Work out the finished part from the listing and answer in its coordinate system (mm). A direction names the side the tool comes from. Give positions to 0.01 mm unless a question says otherwise; leave off trailing zeros. Write each loop counter-clockwise with the first axis right and the second up, starting at its lowest first coordinate (ties: lowest second). Pieces come first, ordered by that corner, then holes.
1) Determine the mould class of faces 5 (the face through (20.35, 0, -14)), 6 (the face through (16, 5, 0.5)), 7 (the face through (0.1, -7, 0.5)) for opening direction Y: pulls with the +Y half, pulls with the -Y half, needs draft (parallel to the pull), parting line crosses it, or undercut.
2) A tool of negligible diameter and unlimited length cuts with its end or side. For faces 1 (the face through (19.065, 0.07, -0.301)), 2 (the face through (-16, -5, 0.5)), 3 (the face through (15.8, -5, 0.5)), 4 (the face through (-10.5, -1.5, 0.5)), from which of +Z, -Z, +X, -X, +Y, -Y can it reach the whole face along a straight path? Write none if from no direction.
3) Find section A-A (z = -5.5). Determine the outline of the cut face in (x, y), plus the area to 3 significant figures.
4) Find section B-B (y = 0). Count the separate pieces of the cut face and the enclosed holes in it, plus the area to 3 significant figures.
5) Find section D-D (x = -5). Determine the outline of the cut face in (y, z).
6) Straight lines are drawn through the part: probe 1 along Y at (x, z) = (20, -25); probe 2 along X at (y, z) = (1.75, -18.75); probe 3 along Z at (x, y) = (4.5, 9). For each, find the intervals that lie inside material, in ascending order.
7) Given pin 1 Ø3.5 at (x, y) = (0, 0) entering from +Z; pin 2 Ø0.8 at (x, z) = (-15.5, 0.5) entering from +Y; pin 3 Ø4 at (y, z) = (0, -25) entering from -X; pin 4 Ø3 at (x, y) = (-1, -7.5) entering from -Z, each flat-ended and moving along its own axis, determine where each tip first touches the part or whether it passes through.
8) Find section C-C (x = 0). Determine the outline of the cut face in (y, z).
```python
from build123d import *

# Parameters (mm, degrees)
SKETCH1_R           = 3
BOSS_EXTRUDE1_DEPTH = 1
SKETCH2_R           = 1.3
BOSS_EXTRUDE2_DEPTH = 1
FILLET1_R           = 1
CUT_EXTRUDE1_DEPTH  = 1


with BuildPart() as part:
    # Sketch1 → Boss-Extrude1 (new body)
    with BuildSketch(Plane.XY):
        with BuildLine():
            ThreePointArc((11.456439237, 5), (0, 12.5), (-11.456439237, 5))
            Line((-11.456439237, 5), (11.456439237, 5))
        make_face()
        with BuildLine():
            Line((11.456439237, 5), (-11.456439237, 5))
            ThreePointArc((-11.456439237, 5), (-12.5, 0), (-11.456439237, -5))
            Line((-11.456439237, -5), (11.456439237, -5))
            ThreePointArc((11.456439237, -5), (12.236328912, -2.553870546), (12.5, 0))
            ThreePointArc((12.5, 0), (12.236328912, 2.553870546), (11.456439237, 5))
        make_face()
        Circle(SKETCH1_R, mode=Mode.SUBTRACT)
        with BuildLine():
            Line((20.35, 5), (11.456439237, 5))
            ThreePointArc((11.456439237, 5), (12.236328912, 2.553870546), (12.5, 0))
            ThreePointArc((12.5, 0), (12.236328912, -2.553870546), (11.456439237, -5))
            Line((11.456439237, -5), (20.35, -5))
            Line((20.35, -5), (20.35, 5))
        make_face()
        with BuildLine():
            Line((-11.456439237, 5), (-20.35, 5))
            Line((-20.35, 5), (-20.35, -5))
            Line((-20.35, -5), (-11.456439237, -5))
            ThreePointArc((-11.456439237, -5), (-12.5, 0), (-11.456439237, 5))
        make_face()
        with BuildLine():
            Line((11.456439237, -5), (-11.456439237, -5))
            ThreePointArc((-11.456439237, -5), (0, -12.5), (11.456439237, -5))
        make_face()
    extrude(amount=BOSS_EXTRUDE1_DEPTH)

    # Sketch2 → Boss-Extrude2 (add)
    with BuildSketch(Plane.ZY.offset(20.35)):
        with BuildLine():
            Line((-25, -3), (0, -5))
            Line((0, -5), (0, 5))
            Line((0, 5), (-25, 3))
            ThreePointArc((-25, 3), (-28, 0), (-25, -3))
        make_face()
        with Locations((-25, 0)):
            Circle(SKETCH2_R, mode=Mode.SUBTRACT)
    boss_extrude2 = extrude(amount=-BOSS_EXTRUDE2_DEPTH)

    # Mirror1: Boss-Extrude2 across plane
    add(boss_extrude2.mirror(Plane.ZY))

    # Fillet1
    fillet1_edges = [part.edges().sort_by_distance(p)[0] for p in [
        (20.35, 0, 1),
        (-20.35, 0, 1),
        (19.35, 0, 0),
        (-19.35, 0, 0),
    ]]
    fillet(fillet1_edges, radius=FILLET1_R)

    # Sketch3 → Cut-Extrude1 (cut)
    with BuildSketch(Plane.XY.offset(1)):
        with BuildLine():
            ThreePointArc((8, 1.5), (6.5, 0), (8, -1.5))
            Line((8, -1.5), (13, -1.5))
            ThreePointArc((13, -1.5), (14.5, 0), (13, 1.5))
            Line((13, 1.5), (8, 1.5))
        make_face()
        with BuildLine():
            ThreePointArc((-4.117647107, 5.660828765), (-1.9e-08, 7), (4.117647076, 5.660828787))
            ThreePointArc((4.117647076, 5.660828787), (6.213034752, 5.991510614), (5.882352933, 8.086898291))
            ThreePointArc((5.882352933, 8.086898291), (6e-09, 10), (-5.882352923, 8.086898298))
            ThreePointArc((-5.882352923, 8.086898298), (-6.213034767, 5.991510634), (-4.117647107, 5.660828765))
        make_face()
        with BuildLine():
            ThreePointArc((4.117647035, -5.660828817), (-2.5e-08, -7), (-4.117647076, -5.660828787))
            ThreePointArc((-4.117647076, -5.660828787), (-6.213034774, -5.991510645), (-5.882352871, -8.086898336))
            ThreePointArc((-5.882352871, -8.086898336), (7.8e-08, -10), (5.882352997, -8.086898245))
            ThreePointArc((5.882352997, -8.086898245), (6.213034714, -5.991510562), (4.117647035, -5.660828817))
        make_face()
        with BuildLine():
            ThreePointArc((-8, -1.5), (-6.5, 0), (-8, 1.5))
            Line((-8, 1.5), (-13, 1.5))
            ThreePointArc((-13, 1.5), (-14.5, 0), (-13, -1.5))
            Line((-13, -1.5), (-8, -1.5))
        make_face()
    extrude(amount=-CUT_EXTRUDE1_DEPTH, mode=Mode.SUBTRACT)


solid = part.part
```
Results:
1. face 5: needs draft
1. face 6: pulls with the +Y half
1. face 7: undercut
2. face 1: -Z, +Y, -Y
2. face 2: +Z, -Z, -X, -Y
2. face 3: +Z, -Z, +X, -Y
2. face 4: +Z, -Z
3. outline: (-20.35, -4.56) - (-19.35, -4.56) - (-19.35, 4.56) - (-20.35, 4.56) - close; (19.35, -4.56) - (20.35, -4.56) - (20.35, 4.56) - (19.35, 4.56) - close
3. area: 18.2 mm2
4. separate pieces: 6
4. enclosed holes: 0
4. area: 69.5 mm2
5. outline: (-11.46, 0) - (-8.66, 0) - (-8.66, 1) - (-11.46, 1) - close; (-5.37, 0) - (5.37, 0) - (5.37, 1) - (-5.37, 1) - close; (8.66, 0) - (11.46, 0) - (11.46, 1) - (8.66, 1) - close
6. probe 1: y = -3 to -1.3, 1.3 to 3
6. probe 2: x = -20.35 to -19.35, 19.35 to 20.35
6. probe 3: z = 0 to 1
7. pin 1: passes through
7. pin 2: stops at y = 5
7. pin 3: stops at x = -20.35
7. pin 4: stops at z = 0
8. outline: (-12.5, 0) - (-10, 0) - (-10, 1) - (-12.5, 1) - close; (-7, 0) - (-3, 0) - (-3, 1) - (-7, 1) - close; (3, 0) - (7, 0) - (7, 1) - (3, 1) - close; (10, 0) - (12.5, 0) - (12.5, 1) - (10, 1) - close
